Build history of the part. All positions in model axes, mm. A direction names the side the tool comes from. Give positions to 0.01 mm unless a question says otherwise; leave off trailing zeros. Loops run counter-clockwise (first coordinate to the right, second up) from the corner with the lowest first, then second, coordinate; pieces in that order, holes last. Notation, with made-up numbers: (32.5, 26.25) - (86.5, 26.25) arc R28 cw to (86.5, 53.25) - close; hole circle Ø6 at (-21.5, -23.75). An arc over 180 degrees is marked (long way). Return JSON: item names as keys, results as strings. Group by question number.
1) Slice it at B-B (z = 13). List the corners of the cut face in (x, y).
2) Mould opens along Z. For faces 3 (the face through (1.09, 25.66, 16.42)), 4 (the face through (17.1, 26.2, 0)), 5 (the face through (17, 26, 15)) say: released by +Z, released by -Z, zero draft, split by the parting line, or undercut.
3) Drill centre lines: probe 1 along X at (y, z) = (18, 2.5); probe 2 along Y at (x, z) = (27.5, 9.5); probe 3 along X at (y, z) = (25.75, 28). Where is each one in solid material? Low to high. Write a range as from..to.
4) Slice it at C-C (y = 10.25). List the corners of the cut face in (x, z), and give its area (3 significant figures).
5) 3-axis set-ups, long thin cutter, end or side, ignore diameter. For faces 1 (the face through (33.1, 29.14, 14.79)), 2 (the face through (4.255, 25.906, 14.79)): which of +Z, -Z, +X, -X, +Y, -Y reach the whole face in a straight line?
6) Slice it at D-D (x = 11.5). List the corners of the cut face in (y, z), and give its area (3 significant figures).
7) Slice it at A-A (y = 2.75). List the corners of the cut face in (x, z).
8) Drop flat-ended pins along their axis: pin 1 (5 mm diameter, centred on x = 21.5, z = 7, fed in from -Y); pin 2 (15 mm diameter, centred on y = 13.07, z = 14.76, fed in from -X) (3 decimals). Give the stop position or say it passes through.
```python
from build123d import *

# Parameters (mm, degrees)
BOSS_EXTRU_1_DEPTH = 30
PER_AGE1_D         = 25.4


with BuildPart() as part:
    # Esquisse1 → Boss.-Extru.1 (new body)
    with BuildSketch(Plane.XY):
        with BuildLine():
            Line((0, 0), (0, 27))
            ThreePointArc((0, 27), (0.878679656, 29.121320344), (3, 30))
            Line((3, 30), (31, 30))
            ThreePointArc((31, 30), (33.121320344, 29.121320344), (34, 27))
            Line((34, 27), (34, 0))
            Line((34, 0), (32, 0))
            Line((32, 0), (32, 23))
            ThreePointArc((32, 23), (31.121320344, 25.121320344), (29, 26))
            Line((29, 26), (5, 26))
            ThreePointArc((5, 26), (2.878679656, 25.121320344), (2, 23))
            Line((2, 23), (2, 0))
            Line((2, 0), (0, 0))
        make_face()
    extrude(amount=BOSS_EXTRU_1_DEPTH)

    # Perçage1 (through all)
    with Locations(Plane.ZY):
        with Locations((14.764081533, 13.067128835)):
            Hole(PER_AGE1_D / 2)


solid = part.part
```
Results:
{
 "1": {"outline": "(0, 0) - (2, 0) - (2, 0.49) - (0, 0.49) - close; (0, 25.64) - (3.58, 25.64) arc R3 cw to (5, 26) - (29, 26) arc R3 cw to (30.42, 25.64) - (34, 25.64) - (34, 27) arc R3 ccw to (31, 30) - (3, 30) arc R3 ccw to (0, 27) - close; (32, 0) - (34, 0) - (34, 0.49) - (32, 0.49) - close"},
 "2": {"face 3": "undercut", "face 4": "released by -Z", "face 5": "zero draft"},
 "3": {"probe 1": "0..2, 32..34", "probe 2": "26..30", "probe 3": "0..3.8, 30.2..34"},
 "4": {"outline": "(0, 0) - (2, 0) - (2, 2.38) - (0, 2.38) - close; (0, 27.15) - (2, 27.15) - (2, 30) - (0, 30) - close; (32, 0) - (34, 0) - (34, 2.38) - (32, 2.38) - close; (32, 27.15) - (34, 27.15) - (34, 30) - (32, 30) - close", "area": "20.9 mm2"},
 "5": {"face 1": "+Z, -Z, +X, +Y", "face 2": "+Z, -Z, -Y"},
 "6": {"outline": "(26, 0) - (30, 0) - (30, 30) - (26, 30) - close", "area": "120 mm2"},
 "7": {"outline": "(0, 0) - (2, 0) - (2, 7.36) - (0, 7.36) - close; (0, 22.17) - (2, 22.17) - (2, 30) - (0, 30) - close; (32, 0) - (34, 0) - (34, 7.36) - (32, 7.36) - close; (32, 22.17) - (34, 22.17) - (34, 30) - (32, 30) - close"},
 "8": {"pin 1": "y = 26", "pin 2": "through"}
}
